Autodesk Inventor part; units mm, degrees
ref_plane "YZ Plane" through (0, 0, 0) normal (1, 0, 0) x (0, 1, 0)
ref_plane "XZ Plane" through (0, 0, 0) normal (0, 1, 0) x (-1, 0, 0)
ref_plane "XY Plane" through (0, 0, 0) normal (0, 0, 1) x (1, 0, 0)
sketch "Sketch1" plane through (0, 0, 0) normal (0, 1, 0) x (-1, 0, 0)
  line L0 (0, 0) -> (0, 10)
  line L1 (0, 10) -> (42.6685, 10)
  line L2 (0, 0) -> (38.0054, 0)
  line L3 (41.8356, -1.7861) -> (53.8302, -16.0807)
  line L4 (55, -19.2946) -> (55, -24.3923)
  line L5 (60, -29.3923) -> (60, -29.3923)
  line L6 (65, -24.3923) -> (65, -15.6549)
  line L7 (63.8302, -12.441) -> (46.4987, 8.2139)
  arc A0 (45.5995, 9.2856) -> (44.0674, 10) centre (44.0674, 8) ccw
  arc A1 (41.8356, -1.7861) -> (38.0054, 0) centre (38.0054, -5) ccw
  arc A2 (55, -19.2946) -> (53.8302, -16.0807) centre (50, -19.2946) ccw
  arc A3 (65, -15.6549) -> (63.8302, -12.441) centre (60, -15.6549) ccw
  arc A4 (46.4987, 8.2139) -> (42.6685, 10) centre (42.6685, 5) ccw
  arc A5 (60, -29.3923) -> (65, -24.3923) centre (60, -24.3923) ccw
  arc A6 (55, -24.3923) -> (60, -29.3923) centre (60, -24.3923) ccw
  point P0 (55, -29.3923)
  point P1 (65, -29.3923)
  point P2 (45, 10)
  point P3 (60, -29.3923)
  dimension "d1" = 130
  dimension "d2" = 140
  dimension "d3" = 45
  dimension "d4" = 20
  dimension "d5" = 10
  dimension "d6" = 10
  dimension "d7" = 10
  dimension "d8" = 2
  dimension "d9" = 5
extrude "Extrusion1" add sketch "Sketch1" along normal blind 3
sketch "Sketch2" plane through (0, 3, 0) normal (0, 1, 0) x (1, 0, 0)
  line L0 (0, -10) -> (0, 0)
  line L1 (0, -5) -> (-25.3234, -5) construction
  arc A0 (-55, 24.3923) -> (-65, 24.3923) centre (-60, 24.3923) ccw
  point P0 (-6.55, -5)
  dimension "d19" = 6.55
hole "Hole1" at (-6.55, 3, 5) at (-60, 3, -24.3923) direction (0, -1, 0) diameter 3.2 end through all
mirror "Mirror1" about plane through (0, 0, 0) normal (1, 0, 0) of "Extrusion1", "Hole1"
properties part number "Claw1" material "Copper, Cast"
The listing builds one solid part. Answer for the finished solid, in the listing's coordinates (mm). A direction names the side the tool comes from. Coordinates: 2 decimals unless noted, no trailing zeros. Loops run counter-clockwise (first coordinate to the right, second up) from the corner with the lowest first, then second, coordinate; pieces in that order, holes last. Notation, with made-up numbers: (82, 10) -> (117, 10) arc R12 cw to (117, 32) -> close; hole circle Ø7 at (61, -1.5). An arc over 180 degrees is marked (long way). Return JSON: item names as keys, results as strings. Group by question number.
(1) Determine the mould class of faces 3 (the cylindrical face through (58.65, 1.48, -23.53)), 4 (the cylindrical face through (-60.11, 1.48, -29.39)), 5 (the cylindrical face through (-44.754, 1.479, 9.544)), 6 (the cylindrical face through (4.964, 1.479, 4.792)) for opening direction Z: released by +Z, released by -Z, zero draft, split by the parting line, or undercut.
(2) A cutting plane is placed at D-D on z = 5. Write down the section's boundary in (x, y).
(3) A cutting plane is placed at A-A on y = 1.4. Write down the section's boundary in (x, z).
(4) A cutting plane is placed at B-B on z = -7. Write down the section's boundary in (x, y), and give its area (3 significant figures).
(5) Which of the six approach directions +Z, -Z, +X, -X, +Y, -Y give full straight-line access (tool end or side, diameter ignored) to faces 1 (the flat face through (55.043, 1.479, -1.969)), 2 (the flat face through (55, 1, -22))?
(6) Find the intervals of material crossed by probe 1 along X at (y, z) = (1.9, 5); probe 2 along Z at (x, y) = (6.55, 1.35); probe 3 along X at (y, z) = (0.15, 5.5), in increasing order. Write a range as from..to.
(7) Given pin 1 Ø4 at (x, z) = (-50, -1.5) entering from -Y; pin 2 Ø1 at (y, z) = (2.5, 6) entering from +X; pin 3 Ø1 at (x, y) = (6.5, 0.5) entering from -Z, each flat-ended and moving along its own axis, determine where each tip first touches the part or whether it passes through.
(8) A cutting plane is placed at C-C on x = 6.55. Write down the section's boundary in (y, z), and give its area (3 significant figures).
The answers:
{
 "1": {"face 3": "undercut", "face 4": "released by -Z", "face 5": "released by +Z", "face 6": "undercut"},
 "2": {"outline": "(-49.2, 0) -> (-8.15, 0) -> (-8.15, 3) -> (-49.2, 3) -> close; (-4.95, 0) -> (4.95, 0) -> (4.95, 3) -> (-4.95, 3) -> close; (8.15, 0) -> (49.2, 0) -> (49.2, 3) -> (8.15, 3) -> close"},
 "3": {"outline": "(-65, -24.39) arc R5 ccw to (-55, -24.39) -> (-55, -19.29) arc R5 cw to (-53.83, -16.08) -> (-41.84, -1.79) arc R5 cw to (-38.01, 0) -> (38.01, 0) arc R5 cw to (41.84, -1.79) -> (53.83, -16.08) arc R5 cw to (55, -19.29) -> (55, -24.39) arc R5 ccw to (65, -24.39) -> (65, -15.65) arc R5 ccw to (63.83, -12.44) -> (46.5, 8.21) arc R5 ccw to (42.67, 10) -> (-42.67, 10) arc R5 ccw to (-46.5, 8.21) -> (-63.83, -12.44) arc R5 ccw to (-65, -15.65) -> close; hole circle Ø3.2 at (-60, -24.39); hole circle Ø3.2 at (-6.55, 5); hole circle Ø3.2 at (6.55, 5); hole circle Ø3.2 at (60, -24.39)"},
 "4": {"outline": "(-59.26, 0) -> (-46.21, 0) -> (-46.21, 3) -> (-59.26, 3) -> close; (46.21, 0) -> (59.26, 0) -> (59.26, 3) -> (46.21, 3) -> close", "area": "78.3 mm^2"},
 "5": {"face 1": "+Z, +X, +Y, -Y", "face 2": "-Z, +Y, -Y"},
 "6": {"probe 1": "x = -49.2..-8.15, -4.95..4.95, 8.15..49.2", "probe 2": "z = 0..3.4, 6.6..10", "probe 3": "x = -48.78..-8.07, -5.03..5.03, 8.07..48.78"},
 "7": {"pin 1": "stops at y = 0", "pin 2": "stops at x = 48.78", "pin 3": "stops at z = 0"},
 "8": {"outline": "(0, 0) -> (3, 0) -> (3, 3.4) -> (0, 3.4) -> close; (0, 6.6) -> (3, 6.6) -> (3, 10) -> (0, 10) -> close", "area": "20.4 mm^2"}
}
